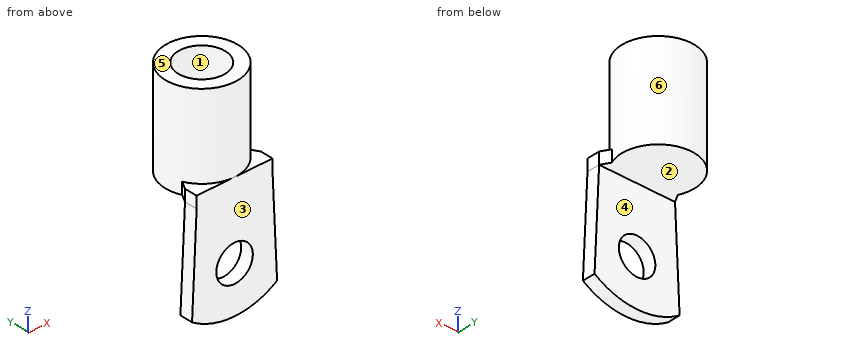
from build123d import *

# Parameters (mm, degrees)
SKETCH1_R                   = 3.96875
LUG_DEPTH                   = 2.794
SKETCH2_R                   = 7.874
SKETCH2_R_2                 = 5.08
CRIMP_SOCKET_DEPTH          = 20.7518
LUG_SOCKET_CONNECTION_DEPTH = 2.54


with BuildPart() as part:
    # Sketch1 → Lug (new body)
    with BuildSketch(Plane(origin=(0, 0, 0), x_dir=(1, 0, 0), z_dir=(0, 1, 0))):
        with BuildLine():
            Line((-9.2456, 7.328412943), (-8.255, -13.97))
            Line((-8.255, -13.97), (8.255, -13.97))
            Line((8.255, -13.97), (9.2456, 7.328412943))
            ThreePointArc((9.2456, 7.328412943), (0, 10.16), (-9.2456, 7.328412943))
        make_face()
        Circle(SKETCH1_R, mode=Mode.SUBTRACT)
    extrude(amount=LUG_DEPTH)

    # Sketch2 → Crimp Socket (add)
    with BuildSketch(Plane.XY.offset(13.97)):
        with Locations((0, 7.874)):
            Circle(SKETCH2_R)
        with Locations((0, 7.874)):
            Circle(SKETCH2_R_2, mode=Mode.SUBTRACT)
    extrude(amount=CRIMP_SOCKET_DEPTH)

    # Sketch3 → Lug Socket Connection (add)
    with BuildSketch(Plane.XY.offset(13.97)):
        with BuildLine():
            Line((8.255, 2.794), (7.183591408, 4.649734117))
            ThreePointArc((7.183591408, 4.649734117), (0, 15.748), (-7.183591408, 4.649734117))
            Line((-7.183591408, 4.649734117), (-8.255, 2.794))
            Line((-8.255, 2.794), (-8.255, 0))
            Line((-8.255, 0), (8.255, 0))
            Line((8.255, 0), (8.255, 2.794))
        make_face()
    extrude(amount=LUG_SOCKET_CONNECTION_DEPTH)


solid = part.part
Geometry: final body of the model. Coordinates: model frame, mm. Face numbers are marked on the shaded views. A direction names the side the tool comes from. Give positions to 0.01 mm unless a question says otherwise; leave off trailing zeros. Write each loop counter-clockwise with the first axis right and the second up, starting at its lowest first coordinate (ties: lowest second). Pieces come first, ordered by that corner, then holes. Notation, with made-up numbers: M -30.5,89 L 0.5,89 A20 ccw 0.5,104 Z; hole C 17.5,24.25 d9. An arc over 180 degrees is marked long. Answer in a Markdown table with one row per item. Add a question column.
(1) Ray query, line 1 (Z direction, x = 0, y = 0.65); line 2 (Y direction, x = 0, z = 31); line 3 (Y direction, x = -6.5, z = 1.5). Return the intervals inside material, ascending.
(2) Section C-C on x = -6. Return loops of the section in (y, z) (3 decimals), and give its area (3 significant figures).
(3) Mould query, pull axis Y, two halves, no side actions, for the marked faces 1, 2, 3 and 4. Classes: +Y half, -Y half, draft (parallel to the pull), parting line (faces both ways), or undercut.
(4) Section A-A on z = -0.5. Return loops of the section in (x, y).
(5) First-contact query: pin 1 (1 mm diameter, centred on x = -1, y = 4, fed in from +Z); pin 2 (10 mm diameter, centred on x = -6.5, z = -3, fed in from +Y); pin 3 (3 mm diameter, centred on y = 1.5, z = 15, fed in from -X); pin 4 (3.5 mm diameter, centred on x = -5, y = 1.5, fed in from +Z). Flat tips, straight axial feed; report the tip coordinate or a pass-through.
(6) Section D-D on z = 16. Return loops of the section in (x, y) (3 decimals), and give its area (3 significant figures).
(7) Section B-B on y = 3.5. Return loops of the section in (x, z), and give its area (3 significant figures).
(8) Reachability of the marked faces 5 and 6 from +Z, -Z, +X, -X, +Y, -Y: full face, straight path, thin tool, end or side. Return the list, or none.
Result set:
| question | item | result |
|---|---|---|
| 1 | line 1 | z = -10.16 to -3.97, 3.97 to 34.72 |
| 1 | line 2 | y = 0 to 2.79, 12.95 to 15.75 |
| 1 | line 3 | y = 0 to 2.79 |
| 2 | outline | M 0,-9.031 L 2.794,-9.031 L 2.794,13.97 L 12.973,13.97 L 12.973,34.722 L 2.775,34.722 L 2.775,16.51 L 0,16.51 Z |
| 2 | area | 283 mm^2 |
| 3 | face 1 | undercut |
| 3 | face 2 | draft |
| 3 | face 3 | -Y half |
| 3 | face 4 | +Y half |
| 4 | outline | M -8.93,0 L -3.94,0 L -3.94,2.79 L -8.93,2.79 Z; M 3.94,0 L 8.93,0 L 8.93,2.79 L 3.94,2.79 Z |
| 5 | pin 1 | stops at z = 16.51 |
| 5 | pin 2 | stops at y = 2.79 |
| 5 | pin 3 | stops at x = -8.28 |
| 5 | pin 4 | stops at z = 34.72 |
| 6 | outline | M -8.255,0 L 8.255,0 L 8.255,2.794 L 7.184,4.65 A7.874 ccw long -7.184,4.65 L -8.255,2.794 Z |
| 6 | area | 221 mm^2 |
| 7 | outline | M -7.85,13.97 L 7.85,13.97 L 7.85,16.51 L 6.55,16.51 L 6.55,34.72 L 2.58,34.72 L 2.58,16.51 L -2.58,16.51 L -2.58,34.72 L -6.55,34.72 L -6.55,16.51 L -7.85,16.51 Z |
| 7 | area | 184 mm^2 |
| 8 | face 5 | +Z, +X, -X, +Y, -Y |
| 8 | face 6 | +Z |
